```python
from build123d import *

# Parameters (mm, degrees)
F2_DEPTH = 329


with BuildPart() as f2:
    # F1 (on Top) → F2 (new body)
    with BuildSketch(Plane.XY):
        with BuildLine():
            Line((34.686533, 111), (-34.686533, 111))
            Line((-34.686533, 111), (-34.686533, 10.5))
            ThreePointArc((-34.686533, 10.5), (0, -24.186533), (34.686533, 10.5))
            Line((34.686533, 10.5), (34.686533, 111))
        make_face()
        with BuildLine():
            Line((-31.686533, 10.5), (-31.686533, 108))
            Line((-31.686533, 108), (31.686533, 108))
            Line((31.686533, 108), (31.686533, 10.5))
            ThreePointArc((31.686533, 10.5), (0, -21.186533), (-31.686533, 10.5))
        make_face(mode=Mode.SUBTRACT)
    extrude(amount=F2_DEPTH)


solid = f2.part
```
Source: CAD feature listing. Evaluate the final solid. Frame: model axes, mm. A direction names the side the tool comes from. Round coordinates to 2 decimals unless told otherwise and drop trailing zeros. Order: outer loops, then holes, each group sorted by start corner. A loop starts at its lowest first (then second) coordinate and runs counter-clockwise, first axis right, second up. Notation, with made-up numbers: (87, -27) -> (91, -27) arc R15 cw to (91, -19) -> close; hole circle Ø7 at (85, 86.5). An arc over 180 degrees is marked (long way). One line per item, written item: value. Start each with the question number.
Q1. Material intervals for probe 1 along X at (y, z) = (18.5, 78); probe 2 along Y at (x, z) = (-23, 187); probe 3 along Y at (x, z) = (6.5, 96.5), sorted ascending.
Q2. Section query A-A (x = 0). Return the cut outline in (y, z), plus the area to 3 significant figures.
Q3. Section query C-C (y = 87.5). Return the cut outline in (x, z), plus the area to 3 significant figures.
Q4. Pin query (flat end, axial travel): pin 1 (10 mm diameter, centred on x = -24.5, z = 64, fed in from -Y); pin 2 (8 mm diameter, centred on y = -3.5, z = 144.5, fed in from +X); pin 3 (3 mm diameter, centred on x = -24, z = 292.5, fed in from -Y). Return the tip coordinate at first contact, or that it passes through.
Q5. Draft query along Y for faces 1 (the flat face through (34.687, 60, 162)), 2 (the flat face through (-31.687, 59, 162)), 3 (the flat face through (0, 111, 162)). Return one class per face: pulls with the +Y half, pulls with the -Y half, needs draft (parallel to the pull), parting line crosses it, or undercut.
Q6. Section query B-B (z = 81.5). Return the cut outline in (x, y).
Q7. Access query for faces 4 (the cylindrical face through (-0.76, -24.18, 162.2)), 5 (the cylindrical face through (0.7, -21.18, 162.2)). Directions: +Z, -Z, +X, -X, +Y, -Y. A direction counts if a zero-diameter tool reaches every point of the face in a straight line with its end or side. Return the directions, or none.
Findings below:
1. probe 1: -34.69 to -31.69, 31.69 to 34.69
1. probe 2: -15.46 to -11.3, 108 to 111
1. probe 3: -23.57 to -20.51, 108 to 111
2. outline: (-24.19, 0) -> (-21.19, 0) -> (-21.19, 329) -> (-24.19, 329) -> close; (108, 0) -> (111, 0) -> (111, 329) -> (108, 329) -> close
2. area: 1,970 mm²
3. outline: (-34.69, 0) -> (-31.69, 0) -> (-31.69, 329) -> (-34.69, 329) -> close; (31.69, 0) -> (34.69, 0) -> (34.69, 329) -> (31.69, 329) -> close
3. area: 1,970 mm²
4. pin 1: y = -18.19
4. pin 2: x = 33.21
4. pin 3: y = -15.9
5. face 1: needs draft
5. face 2: undercut
5. face 3: pulls with the +Y half
6. outline: (-34.69, 10.5) arc R34.69 ccw to (34.69, 10.5) -> (34.69, 111) -> (-34.69, 111) -> close; hole (-31.69, 10.5) arc R31.69 ccw to (31.69, 10.5) -> (31.69, 108) -> (-31.69, 108) -> close
7. face 4: +Z, -Z, -Y
7. face 5: +Z, -Z
